Build history of the part. All positions in model axes, mm. A direction names the side the tool comes from. Round coordinates to 2 decimals unless told otherwise and drop trailing zeros. Order: outer loops, then holes, each group sorted by start corner. A loop starts at its lowest first (then second) coordinate and runs counter-clockwise, first axis right, second up. Notation, with made-up numbers: M -23.5,78 L -1.5,78 A10 cw -1.5,96 Z; hole C -9,-40 d9. An arc over 180 degrees is marked long. One line per item, written item: value. Start each with the question number.
Item 1: Tool access for faces 1 (the flat face through (-1, -5.2, 5.2)), 2 (the cylindrical face through (-0.49, -11.99, -0.53)): list every direction of +Z, -Z, +X, -X, +Y, -Y with a clear straight run to the whole face (end or side of a thin tool).
Item 2: Band-saw the part on D-D, the plane z = 8.5. Write the cut outline in (x, y).
Item 3: Pin check, flat tip, straight feed: pin 1 (3 mm diameter, centred on y = -4.5, z = -9, fed in from -X). Stop position of the tip, or through.
Item 4: Band-saw the part on C-C, the plane x = -1.75. Write the cut outline in (y, z).
Item 5: Band-saw the part on A-A, the plane z = 0. Write the cut outline in (x, y).
Item 6: Two-plate mould, pull along Z, no slides. Class faces 3 (the cylindrical face through (-1.986, 6.466, 2.681)), 4 (the cylindrical face through (-2, -6, 0)), 5 (the flat face through (-3, -6, -2)): +Z half, -Z half, draft (parallel to the pull), parting line (faces both ways), or undercut.
Item 7: Probe L1, parallel to Z at x = -1.05, y = 0; L2, parallel to X at y = -8.75, z = 4.5. List the from-to ranges inside material, lowest first.
```python
from build123d import *

# Parameters (mm, degrees)
CHAMFER1_SIZE = 0.5


with BuildPart() as part:
    # Sketch1 → Revolve1 (revolve)
    with BuildSketch(Plane.XY):
        Polygon((0, 6), (-1, 6), (-3, 6), (-3, 7), (-1, 7), (-1, 12), (0, 12), align=None)
    revolve(axis=Axis((0, 0, 0), (-1, 0, 0)))

    # Chamfer1
    chamfer1_edges = [part.edges().sort_by_distance(p)[0] for p in [
        (0, -6, 0),
    ]]
    chamfer(chamfer1_edges, length=CHAMFER1_SIZE)


solid = part.part
```
Output:
1. face 1: -X
1. face 2: +X, -X
2. outline: M -1,-8.47 L 0,-8.47 L 0,8.47 L -1,8.47 Z
3. pin 1: stops at x = -1
4. outline: C 0,0 d14; hole C 0,0 d12
5. outline: M -3,-7 L -1,-7 L -1,-12 L 0,-12 L 0,-6.5 L -0.5,-6 L -3,-6 Z; M -3,6 L -0.5,6 L 0,6.5 L 0,12 L -1,12 L -1,7 L -3,7 Z
6. face 3: parting line
6. face 4: undercut
6. face 5: draft
7. L1: z = -7 to -6, 6 to 7
7. L2: x = -1 to 0
